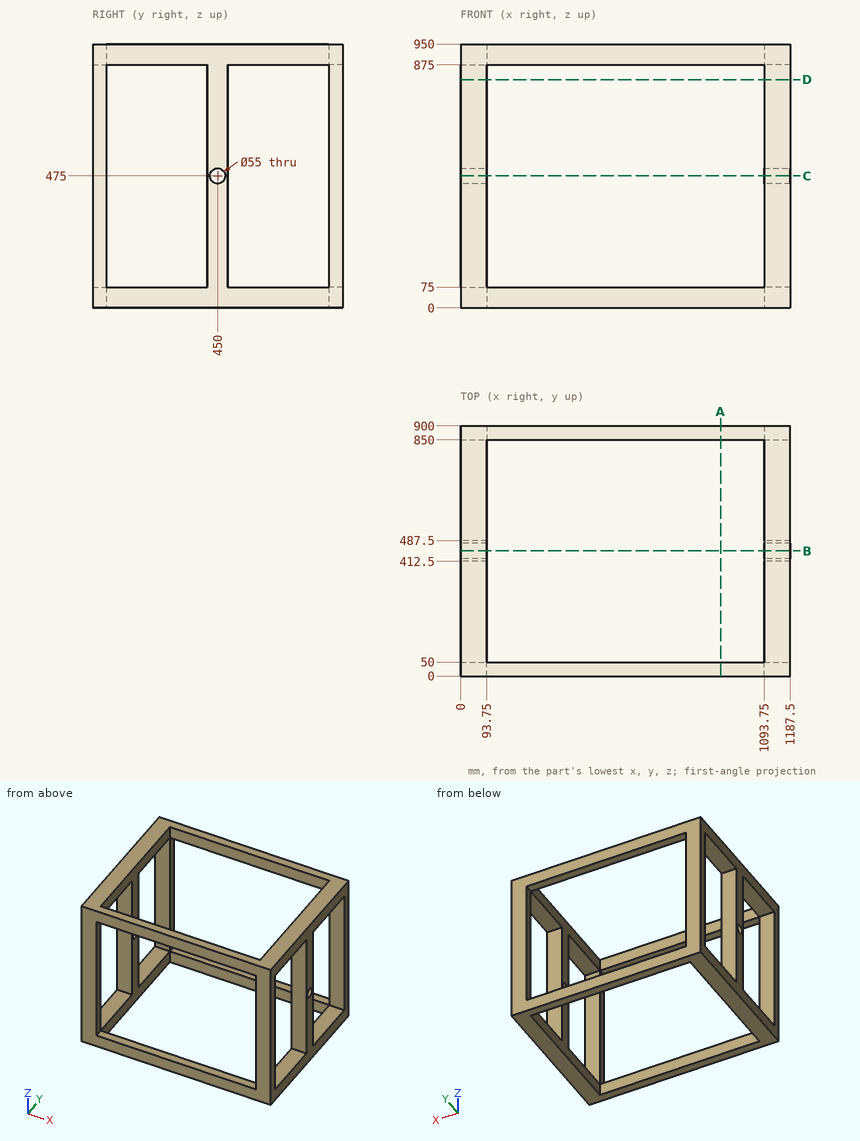
Check sheet for the drawn part. Datum: minimum x, y, z corner. Units: mm. Give positions to 0.01 mm unless a question says otherwise; leave off trailing zeros. Write each loop counter-clockwise with the first axis right and the second up, starting at its lowest first coordinate (ties: lowest second). Pieces come first, ordered by that corner, then holes. Notation, with made-up numbers: (68, 83.25) -> (87, 83.25) arc R7 ccw to (87, 89.25) -> close; hole circle Ø4 at (-1.5, 66.25). An arc over 180 degrees is marked (long way). Use one line per item in the form item = value. Start each with the question number.
1. Section check C-C (z = 475). Count the separate pieces of the cut face and the enclosed holes in it, and give its area (3 significant figures).
2. Thickness scan on line 1 along Y through (x, z) = (1134, 475); line 2 along Y through (x, z) = (1107.5, 513); line 3 along X through (y, z) = (467, 430). Record the ranges inside material, lowest first. Write a range as from..to.
3. Go/stop test with a flat-tipped pin: P1, Ø15, axis at y = 868.5, z = 294.5, coming from the -X side. Record where the tip stops, or that it passes through.
4. Section check A-A (x = 936). Record the cut outline in (y, z), and give its area (3 significant figures).
5. Section check B-B (y = 450). Record the cut outline in (x, z).
6. Section check D-D (z = 822). Record the cut outline in (x, y), and give its area (3 significant figures).
Conclusion:
q1.separate_pieces = 8
q1.enclosed_holes = 0
q1.area = 22,500 mm²
q2.line_1 = 0..50, 412.5..422.5, 477.5..487.5, 850..900
q2.line_2 = 0..50, 412.5..487.5, 850..900
q2.line_3 = 0..93.75, 1093.75..1187.5
q3.P1 = 0
q4.outline = (0, 0) -> (50, 0) -> (50, 75) -> (0, 75) -> close; (0, 875) -> (50, 875) -> (50, 950) -> (0, 950) -> close; (850, 0) -> (900, 0) -> (900, 75) -> (850, 75) -> close; (850, 875) -> (900, 875) -> (900, 950) -> (850, 950) -> close
q4.area = 15,000 mm²
q5.outline = (0, 0) -> (93.75, 0) -> (93.75, 447.5) -> (0, 447.5) -> close; (0, 502.5) -> (93.75, 502.5) -> (93.75, 950) -> (0, 950) -> close; (1093.75, 0) -> (1187.5, 0) -> (1187.5, 447.5) -> (1093.75, 447.5) -> close; (1093.75, 502.5) -> (1187.5, 502.5) -> (1187.5, 950) -> (1093.75, 950) -> close
q6.outline = (0, 0) -> (93.75, 0) -> (93.75, 50) -> (0, 50) -> close; (0, 412.5) -> (93.75, 412.5) -> (93.75, 487.5) -> (0, 487.5) -> close; (0, 850) -> (93.75, 850) -> (93.75, 900) -> (0, 900) -> close; (1093.75, 0) -> (1187.5, 0) -> (1187.5, 50) -> (1093.75, 50) -> close; (1093.75, 412.5) -> (1187.5, 412.5) -> (1187.5, 487.5) -> (1093.75, 487.5) -> close; (1093.75, 850) -> (1187.5, 850) -> (1187.5, 900) -> (1093.75, 900) -> close
q6.area = 32,800 mm²
